Work out the finished part from the listing and answer in its coordinate system (mm). Give positions to 0.01 mm unless a question says otherwise; leave off trailing zeros. Loops run counter-clockwise (first coordinate to the right, second up) from the corner with the lowest first, then second, coordinate; pieces in that order, holes last. Notation, with made-up numbers: M 13,71.25 L 43,71.25 A36 ccw 43,110.25 Z; hole C 19.25,17.5 d7. An arc over 180 degrees is marked long. Use a Markdown table: item, result.
Autodesk Inventor part; units mm, degrees
ref_plane "YZ Plane" through (0, 0, 0) normal (1, 0, 0) x (0, 1, 0)
ref_plane "XZ Plane" through (0, 0, 0) normal (0, 1, 0) x (-1, 0, 0)
ref_plane "XY Plane" through (0, 0, 0) normal (0, 0, 1) x (1, 0, 0)
sketch "Sketch1" plane through (0, 0, 0) normal (0, 1, 0) x (-1, 0, 0)
  line L0 (-4.445, 0) -> (-38.1, 0)
  line L1 (-38.1, -139.7) -> (-4.445, -139.7)
  line L2 (0, -135.255) -> (0, -4.445)
  arc A0 (-55.8268, -134.9145) -> (-55.8268, -4.7855) centre (-166.37, -69.85) ccw
  line L3 (-38.1, 0) -> (-53.0906, 0)
  line L4 (-53.0906, -139.7) -> (-38.1, -139.7)
  arc A1 (-4.445, -139.7) -> (0, -135.255) centre (-4.445, -135.255) ccw
  arc A2 (0, -4.445) -> (-4.445, 0) centre (-4.445, -4.445) ccw
  arc A3 (-53.0906, 0) -> (-55.8268, -4.7855) centre (-53.0906, -3.175) ccw
  arc A4 (-55.8268, -134.9145) -> (-53.0906, -139.7) centre (-53.0906, -136.525) ccw
  circle A5 centre (-6.35, -6.35) radius 2.2225
  circle A6 centre (-6.35, -19.05) radius 2.2225
  circle A7 centre (-6.35, -133.35) radius 2.2225
  circle A8 centre (-6.35, -120.65) radius 2.2225
  point P0 (0, 0)
  point P1 (0, -139.7)
  point P2 (-58.7867, -139.7)
  point P3 (-58.7867, 0)
  dimension "d0" = 38.1
  dimension "d4" = 4.445
  dimension "d5" = 4.445
  dimension "d6" = 3.175
  dimension "d7" = 4.445
  dimension "d8" = 4.445
  dimension "d9" = 4.445
  dimension "d10" = 4.445
extrude "Extrusion1" add sketch "Sketch1" along normal blind 1.778
properties part number "claw_aligner_piece"
(1) A cutting plane is placed at B-B (x = 6.35). Write down the section's boundary in (y, z).
Entries:
| item | result |
|---|---|
| outline | M 0,-139.7 L 1.78,-139.7 L 1.78,-135.57 L 0,-135.57 Z; M 0,-131.13 L 1.78,-131.13 L 1.78,-122.87 L 0,-122.87 Z; M 0,-118.43 L 1.78,-118.43 L 1.78,-21.27 L 0,-21.27 Z; M 0,-16.83 L 1.78,-16.83 L 1.78,-8.57 L 0,-8.57 Z; M 0,-4.13 L 1.78,-4.13 L 1.78,0 L 0,0 Z |
(2) A cutting plane is placed at C-C (z = -6.35). Write down the section's boundary in (x, y).
Entries:
| item | result |
|---|---|
| outline | M 0,0 L 4.13,0 L 4.13,1.78 L 0,1.78 Z; M 8.57,0 L 54.92,0 L 54.92,1.78 L 8.57,1.78 Z |
(3) A cutting plane is placed at D-D (x = 44.5). Write down the section's boundary in (y, z).
Entries:
| item | result |
|---|---|
| outline | M 0,-139.7 L 1.78,-139.7 L 1.78,-109.86 L 0,-109.86 Z; M 0,-29.84 L 1.78,-29.84 L 1.78,0 L 0,0 Z |
(4) A cutting plane is placed at A-A (y = 0.85). Count the separate pieces of the cut face and the enclosed holes in it, and give its area (3 significant figures).
Entries:
| item | result |
|---|---|
| separate pieces | 1 |
| enclosed holes | 4 |
| area | 6,170 mm² |
(5) Consider probe 1 along Z at (x, y) = (6.35, 1.3); probe 2 along Z at (x, y) = (52.5, 0.75); probe 3 along Z at (x, y) = (53, 1.3). Determine where each line is inside the solid, lowest interval first. Write a range as [from, to].
Entries:
| item | result |
|---|---|
| probe 1 | z = [-139.7, -135.57], [-131.13, -122.87], [-118.43, -21.27], [-16.83, -8.57], [-4.13, 0] |
| probe 2 | z = [-139.7, -128.9], [-10.8, 0] |
| probe 3 | z = [-139.7, -129.85], [-9.85, 0] |
(6) The mould has two halves that part along X. Classify faces 1 (the cylindrical face through (55.823, 0.877, -138.141)), 2 (the cylindrical face through (1.337, 0.877, -1.268)), 3 (the cylindrical face through (6.639, 0.877, -122.854)): released by +X, released by -X, zero draft, split by the parting line, or undercut.
Entries:
| item | result |
|---|---|
| face 1 | released by +X |
| face 2 | released by -X |
| face 3 | undercut |
(7) Given P1, Ø2.5, axis at x = 6.35, z = -19.05, coming from the -Y side, flat-ended and moving along its own axis, determine where the tip first touches the part or whether it passes through.
Entries:
| item | result |
|---|---|
| P1 | passes through |
